from build123d import *

# Parameters (mm, degrees)
F0_R     = 10
F1_DEPTH = 1406
F2_R     = 7.5
F3_DEPTH = 1800
F6_DEPTH = 300
F8_R     = 15
F9_DEPTH = 200
F10_SIZE = 4.99999
F11_SIZE = 1
F12_SIZE = 2


# Not quite as in the source:
# - a fillet or chamfer is up to 0.001 mm smaller than in the source, because OpenCascade refuses the exact size
# - a feature names something its author has since deleted; it is built from what else it names


with BuildPart() as f1:
    # F0 (on Front) → F1 (new body)
    with BuildSketch(Plane.XZ):
        Circle(F0_R)
    extrude(amount=-F1_DEPTH)

    # F2 (on Front) → F3 (cut)
    with BuildSketch(Plane.XZ):
        Circle(F2_R)
    extrude(amount=-F3_DEPTH, mode=Mode.SUBTRACT)

    # F5 (on offset) → F6 (join)
    with BuildSketch(Plane.YZ.offset(165)):
        with BuildLine():
            Line((0, 82), (0, -15))
            Line((0, -15), (6, -15))
            Line((6, -15), (6, 82))
            ThreePointArc((6, 82), (3, 85), (0, 82))
        make_face()
    extrude(amount=-F6_DEPTH)

    # F8 (on offset) → F9 (join)
    with BuildSketch(Plane.XZ.offset(-1256)):
        Circle(F8_R)
    extrude(amount=F9_DEPTH)

    # F10 (size 5 in the source; OpenCascade refuses exactly that, so slightly less here)
    f10_edges = [f1.edges().sort_by_distance(p)[0] for p in [
        (15, 1156, 0),
        (-15, 1256, 0),
        (-15, 1056, 0),
    ]]
    chamfer(f10_edges, length=F10_SIZE)

    # F11
    f11_edges = [f1.edges().sort_by_distance(p)[0] for p in [
        (-10, 6, 0),
    ]]
    chamfer(f11_edges, length=F11_SIZE)

    # F12
    f12_edges = [f1.edges().sort_by_distance(p)[0] for p in [
        (165, 0, 33.5),
        (165, 3, -15),
        (165, 6, 33.5),
        (165, 3, 85),
        (15, 0, -15),
        (15, 6, -15),
        (15, 6, 82),
        (-135, 6, 33.5),
        (-135, 0, 33.5),
        (15, 0, 82),
        (-135, 3, 85),
    ]]
    chamfer(f12_edges, length=F12_SIZE)


solid = f1.part
Could you check a few things on this model? Use its own coordinates, in mm. Give positions to 0.01 mm unless a question says otherwise; leave off trailing zeros. Order: outer loops, then holes, each group sorted by start corner. A loop starts at its lowest first (then second) coordinate and runs counter-clockwise, first axis right, second up. Notation, with made-up numbers: (36.5, -14) - (94.5, -14) arc R28 ccw to (94.5, 21) - close; hole circle Ø11 at (-22, 85). An arc over 180 degrees is marked (long way). Return JSON: item names as keys, results as strings. Group by question number.
Q1. Please list where these lines run through material, in increasing order: line 1 along Z through (x, y) = (0, 1309.5); line 2 along Y through (x, z) = (-50, 9.5); line 3 along X through (y, z) = (621.5, 2.5). Write a range as [from, to].
Q2. Suppose I cut it at A-A, the plane y = 121. Please give me the cut outline in (x, z).
Q3. Suppose I cut it at C-C, the plane z = 45.5. Please give me the cut outline in (x, y).
Q4. Thinking about a two-plate mould opening in Y: for faces 1 (the face through (-2.22, 1255.757, -9.999)), 2 (the face through (17, 0, 35)), 3 (the face through (-2.22, 1056.243, -9.999)), 4 (the face through (-14.985, 1157.33, 0.66)), which applies, pulls with the +Y half, pulls with the -Y half, needs draft (parallel to the pull), parting line crosses it, or undercut?
Q5. Will this pin go through, and if not, where does the flat tip stop? pin 1 Ø10 at (x, z) = (33.5, 20.5) entering from +Y.
Q6. Suppose I cut it at B-B, the plane x = 92. Please give me the cut outline in (y, z).
Resolved:
{
 "1": {"line 1": "z = [-10, -7.5], [7.5, 10]", "line 2": "y = [0, 6]", "line 3": "x = [-9.68, -7.07], [7.07, 9.68]"},
 "2": {"outline": "circle Ø20 at (0, 0); hole circle Ø15 at (0, 0)"},
 "3": {"outline": "(-135, 2) - (-133, 0) - (163, 0) - (165, 2) - (165, 4) - (163, 6) - (-133, 6) - (-135, 4) - close"},
 "4": {"face 1": "pulls with the +Y half", "face 2": "pulls with the -Y half", "face 3": "undercut", "face 4": "needs draft"},
 "5": {"pin 1": "stops at y = 6"},
 "6": {"outline": "(0, -13) - (2, -15) - (4, -15) - (6, -13) - (6, 82) arc R3 ccw to (0, 82) - close"}
}
